```python
from build123d import *

# Parameters (mm, degrees)
SKETCH1_R               = 2.200000000000002
SKETCH1_R_2             = 1.6499999999999986
BOSS_EXTRUDE1_DEPTH     = 15.239999999999998
SKETCH2_R               = 4.8260000000000005
CUT_EXTRUDE1_DEPTH      = 3.8099999999999996
FILLET2_R               = 2.54
FILLET3_R               = 3
CUT_EXTRUDE2_DEPTH      = 5
CUT_EXTRUDE2_DEPTH_BACK = 5
FILLET4_R               = 10


with BuildPart() as part:
    # Sketch1 → Boss-Extrude1 (new body)
    with BuildSketch(Plane(origin=(0, 0, 0), x_dir=(1, 0, 0), z_dir=(0, 1, 0))):
        with BuildLine():
            ThreePointArc((11.827375744432914, 8.128), (0, 14.350999999999997), (-11.827375744432915, 8.128))
            Line((-11.827375744432912, 8.128), (-22.270000000000003, 8.127999999999998))
            Line((-22.270000000000003, 8.127999999999998), (-22.270000000000003, 3.8623859206454227))
            ThreePointArc((-22.270000000000003, 3.8623859206454245), (-22.30372167021767, -3.8429822403961222), (-15.625000000000004, -6.7e-16))
            Line((-15.625, 0), (-1.6509999999999998, 0))
            ThreePointArc((-1.651, -4.2e-16), (-3.8e-16, 1.6509999999999998), (1.6509999999999996, 0))
            Line((1.6509999999999998, 0), (14.350999999999999, -1.6e-16))
            Line((14.350999999999999, -1.6e-16), (19.351, 8.7e-16))
            ThreePointArc((19.351, 1.78e-15), (23.351, 4.000000000000002), (19.351, 8.000000000000002))
            Line((19.351, 8.000000000000002), (11.914327551314004, 8))
            ThreePointArc((11.914327551314003, 7.999999999999999), (11.871024170046155, 8.064117196208148), (11.82737574443291, 8.128))
        make_face()
        with Locations(Location((-20.07, 0, 0), (0, 0, 90))):
            Circle(SKETCH1_R, mode=Mode.SUBTRACT)
        with Locations(Location((19.351, 4.000000000000001, 0), (0, 0, 90))):
            Circle(SKETCH1_R_2, mode=Mode.SUBTRACT)
    extrude(amount=BOSS_EXTRUDE1_DEPTH)

    # Sketch2 → Cut-Extrude1 (cut, symmetric)
    with BuildSketch(Plane(origin=(0, 15.239999999999998, 0), x_dir=(1, 0, 0), z_dir=(0, 1, 0))):
        with Locations((-20.07, 0)):
            Circle(SKETCH2_R)
    cut_extrude1 = extrude(amount=CUT_EXTRUDE1_DEPTH, both=True, mode=Mode.SUBTRACT)

    # Fillet2
    fillet2_edges = [part.edges().sort_by_distance(p)[0] for p in [
        (-3.8e-16, 15.239999999999998, -1.6509999999999998),
    ]]
    fillet(fillet2_edges, radius=FILLET2_R)

    # Mirror1: Cut-Extrude1 across plane
    add(cut_extrude1.mirror(Plane.ZX.offset(7.619999999999999)), mode=Mode.SUBTRACT)

    # Fillet3
    fillet3_edges = [part.edges().sort_by_distance(p)[0] for p in [
        (-22.270000000000003, 7.619999999999999, -3.8623859206454227),
    ]]
    fillet(fillet3_edges, radius=FILLET3_R)

    # Sketch3 → Cut-Extrude2 (cut, two sides: drawn at the far end of the back side and taken through both)
    with BuildSketch(Plane(origin=(0, 7.619999999999999, 0), x_dir=(1, 0, 0), z_dir=(0, 1, 0)).offset(-CUT_EXTRUDE2_DEPTH_BACK)):
        with BuildLine():
            Line((14.350999999999999, -1.6e-16), (19.351, 8.7e-16))
            ThreePointArc((19.351, 8.7e-16), (23.351, 4.000000000000001), (19.351, 8))
            Line((19.351, 8), (11.914327551314004, 8))
            ThreePointArc((11.914327551314004, 8), (13.728323198572127, 4.181428363077186), (14.350999999999999, -1.6e-16))
        make_face()
    extrude(amount=CUT_EXTRUDE2_DEPTH + CUT_EXTRUDE2_DEPTH_BACK, mode=Mode.SUBTRACT)

    # Fillet4
    fillet4_edges = [part.edges().sort_by_distance(p)[0] for p in [
        (11.914327551314003, 13.93, -8),
        (11.914327551314003, 1.3099999999999996, -8),
    ]]
    fillet(fillet4_edges, radius=FILLET4_R)


solid = part.part
```
Can you work these out from the model? Positions are in its coordinate system, mm. A direction names the side the tool comes from. Round coordinates to 2 decimals unless told otherwise and drop trailing zeros. Loops run counter-clockwise (first coordinate to the right, second up) from the corner with the lowest first, then second, coordinate; pieces in that order, holes last. Notation, with made-up numbers: M -0.5,-17.75 L 33.5,-17.75 A26 cw 33.5,-0.75 Z; hole C 36,-36 d1. An arc over 180 degrees is marked long. Answer as a JSON object with one key per item and string values. Group by question number.
Q1. We'd pull the mould along X, two halves only. Please class faces 5 (the cylindrical face through (-22.408, 7.727, -4.428)), 6 (the cylindrical face through (-0.04, 6.26, -1.65)), 7 (the cylindrical face through (23.35, 13.91, -3.91)): +X half, -X half, draft (parallel to the pull), parting line (faces both ways), or undercut.
Q2. Will these pins go through, and if not, where does the flat tip stop? pin 1 (2 mm diameter, centred on y = 8.5, z = -6.5, fed in from -X); pin 2 (5 mm diameter, centred on y = 6, z = -2, fed in from +X); pin 3 (5 mm diameter, centred on x = -18, y = 8.5, fed in from -Z).
Q3. Imagine slicing it at D-D, the plane x = 11.5. Please give me the cut outline in (y, z), then the cut area to 3 significant figures.
Q4. Please list where these lines run through material, in increasing order: L1, parallel to Y at x = 20, z = -7.25; L2, parallel to X at y = 14.3, z = -4; L3, parallel to Z at x = -20, y = 11.5.
Q5. Imagine slicing it at C-C, the plane z = -9.5. Please give me the cut outline in (x, y).
Q6. On a 3-axis mill with a long thin cutter (end or side, diameter ignored), from which of +Z, -Z, +X, -X, +Y, -Y can I reach the whole of each face in a straight line? I mean faces 1 (the cylindrical face through (-17.61, 13.36, -4.15)), 2 (the flat face through (18, 1, -8)), 3 (the cylindrical face through (4.498, 7.513, -13.628)), 4 (the flat face through (-22.27, 8, -7)). Say none if no direction works.
Q7. Imagine slicing it at A-A, the plane y = 8. Please give me the cut outline in (x, z) (3 decimals).
Q8. Imagine slicing it at B-B, the plane x = -20.07. Please give me the cut outline in (y, z) (3 decimals), then the cut area to 3 significant figures.
Findings:
{
 "1": {"face 5": "-X half", "face 6": "undercut", "face 7": "+X half"},
 "2": {"pin 1": "stops at x = -22.27", "pin 2": "stops at x = 14.35", "pin 3": "stops at z = -8.13"},
 "3": {"outline": "M 0,-9.28 L 2.62,-9.28 L 2.62,-8.58 L 12.62,-8.58 L 12.62,-9.28 L 15.24,-9.28 L 15.24,0 L 0,0 Z", "area": "134 mm2"},
 "4": {"L1": "y = 0 to 2.62, 12.62 to 15.24", "L2": "x = -17.37 to 17.7, 21 to 23.35", "L3": "z = -8.13 to -4.83"},
 "5": {"outline": "M -10.76,0 L 11.13,0 L 11.13,2.62 L 10.76,2.62 L 10.76,12.62 L 11.13,12.62 L 11.13,15.24 L -10.76,15.24 Z"},
 "6": {"face 1": "+Z, +Y", "face 2": "-Z, +X, +Y, -Y", "face 3": "-Z", "face 4": "-Z, -X, +Y, -Y"},
 "7": {"outline": "M -23.175,-3.181 A3 cw -22.27,-5.328 L -22.27,-8.128 L -11.827,-8.128 A14.351 ccw 14.351,0 L 1.651,0 A1.651 cw -1.651,0 L -15.625,0 A4.445 ccw long Z; hole C -20.07,0 d4.4"},
 "8": {"outline": "M 0,-8.128 L 15.24,-8.128 L 15.24,-4.826 L 11.43,-4.826 L 11.43,-2.2 L 3.81,-2.2 L 3.81,-4.826 L 0,-4.826 Z; M 3.81,2.2 L 11.43,2.2 L 11.43,4.445 L 3.81,4.445 Z", "area": "87.4 mm2"}
}
